Answer from the drawing. Dimensions are ordinates in mm from the lowest x, y and z of the part. A direction names the side the tool comes from. Coordinates: 2 decimals unless noted, no trailing zeros. Write each loop counter-clockwise with the first axis right and the second up, starting at its lowest first coordinate (ties: lowest second). Pieces come first, ordered by that corner, then holes.
(1) For a pull along Z with two mould halves and no side action, classify the marked faces 1, 2, 3 and 4 as +Z half, -Z half, draft (parallel to the pull), parting line (faces both ways), or undercut.
(2) The part is cut by section B-B on y = 6. Determine the outline of the cut face in (x, z), plus the area to 3 significant figures.
(3) Straight lines are drawn through the part: line 1 (Z direction, x = 20.5, y = 5); line 2 (X direction, y = 1, z = 17.5); line 3 (Y direction, x = 15.5, z = 26). For each, find the intervals that lie inside material, in ascending order.
(4) The part is cut by section C-C on z = 4. Determine the outline of the cut face in (x, y).
(5) The part is cut by section D-D on y = 0.75. Determine the outline of the cut face in (x, z), plus the area to 3 significant figures.
(6) The part is cut by section A-A on x = 14.5. Determine the outline of the cut face in (y, z).
(7) Which of the six approach directions +Z, -Z, +X, -X, +Y, -Y give full straight-line access (tool end or side, diameter ignored) to the marked faces 5, 6 and 7?
(8) Given P1, Ø2, axis at x = 20.5, y = 3.5, coming from the +Z side; P2, Ø2, axis at y = 3.5, z = 12, coming from the -X side; P3, Ø2.5, axis at x = 20, z = 26, coming from the -Y side, each flat-ended and moving along its own axis, determine where each tip first touches the part or whether it passes through.
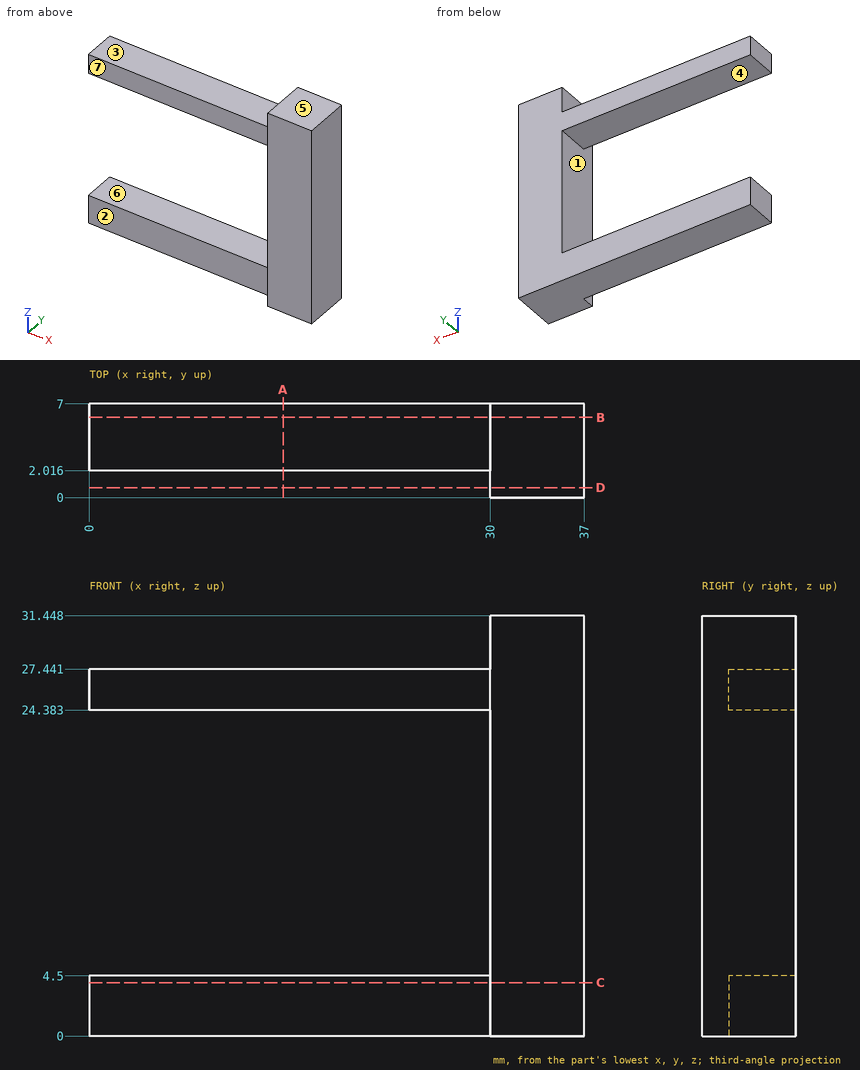
Model answer:
1. face 1: undercut
1. face 2: draft
1. face 3: +Z half
1. face 4: undercut
2. outline: (0, 0) - (37, 0) - (37, 31.45) - (30, 31.45) - (30, 27.44) - (0, 27.44) - (0, 24.38) - (30, 24.38) - (30, 4.5) - (0, 4.5) - close
2. area: 447 mm2
3. line 1: z = 0 to 4.5, 24.38 to 27.44
3. line 2: x = 30 to 37
3. line 3: y = 2.02 to 7
4. outline: (0, 2.02) - (30, 2.02) - (30, 0) - (37, 0) - (37, 7) - (0, 7) - close
5. outline: (30, 0) - (37, 0) - (37, 31.45) - (30, 31.45) - close
5. area: 220 mm2
6. outline: (2.02, 0) - (7, 0) - (7, 4.5) - (2.02, 4.5) - close; (2.02, 24.38) - (7, 24.38) - (7, 27.44) - (2.02, 27.44) - close
7. face 5: +Z, +X, -X, +Y, -Y
7. face 6: -X, +Y, -Y
7. face 7: +Z, -Z, -X, -Y
8. P1: stops at z = 27.44
8. P2: stops at x = 30
8. P3: stops at y = 2.02
